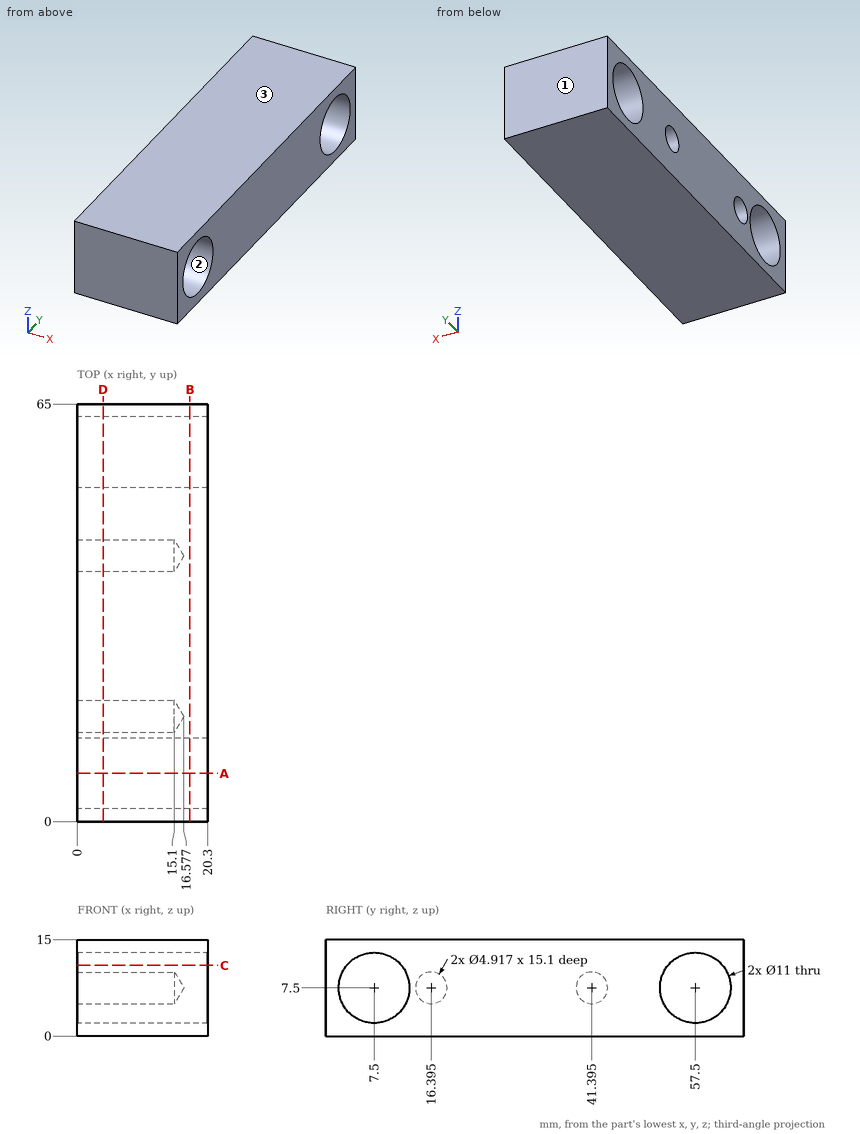
Answer from the drawing. Dimensions are ordinates in mm from the lowest x, y and z of the part. Coordinates: 2 decimals unless noted, no trailing zeros. Loops run counter-clockwise (first coordinate to the right, second up) from the corner with the lowest first, then second, coordinate; pieces in that order, holes last. Notation, with made-up numbers: (69, -1.75) -> (100, -1.75) arc R31 ccw to (100, 25.25) -> close; hole circle Ø2 at (-36.5, 13.5). An arc over 180 degrees is marked (long way). Return JSON: item names as keys, results as strings.
Item 1: Find section D-D (x = 4). Determine the outline of the cut face in (y, z) (1 decimal), plus the area to 3 significant figures.
Answers:
{"outline": "(0, 0) -> (65, 0) -> (65, 15) -> (0, 15) -> close; hole circle Ø11 at (7.5, 7.5); hole circle Ø4.9 at (16.4, 7.5); hole circle Ø4.9 at (41.4, 7.5); hole circle Ø11 at (57.5, 7.5)", "area": "747 mm2"}
Item 2: Find section A-A (y = 7.5). Determine the outline of the cut face in (x, z), plus the area to 3 significant figures.
Answers:
{"outline": "(0, 0) -> (20.3, 0) -> (20.3, 2) -> (0, 2) -> close; (0, 13) -> (20.3, 13) -> (20.3, 15) -> (0, 15) -> close", "area": "81.2 mm2"}
Item 3: Flat-ended cylindrical pins translate along their axes: P1, Ø1, axis at y = 27.5, z = 13, coming from the -X side; P2, Ø6.5, axis at y = 57.5, z = 7.5, coming from the -X side. Find the tip coordinate at first contact, or state that the pin passes through.
Answers:
{"P1": "stops at x = 0", "P2": "passes through"}
Item 4: Find section B-B (x = 17.5). Determine the outline of the cut face in (y, z), plus the area to 3 significant figures.
Answers:
{"outline": "(0, 0) -> (65, 0) -> (65, 15) -> (0, 15) -> close; hole circle Ø11 at (7.5, 7.5); hole circle Ø11 at (57.5, 7.5)", "area": "785 mm2"}
Item 5: Find section C-C (z = 11). Determine the outline of the cut face in (x, y).
Answers:
{"outline": "(0, 0) -> (20.3, 0) -> (20.3, 3.26) -> (0, 3.26) -> close; (0, 11.74) -> (20.3, 11.74) -> (20.3, 53.26) -> (0, 53.26) -> close; (0, 61.74) -> (20.3, 61.74) -> (20.3, 65) -> (0, 65) -> close"}
Item 6: Find the intervals of material crossed by probe 1 along Y at (x, z) = (12.5, 7.5); probe 2 along Y at (x, z) = (12, 10.5); probe 3 along Y at (x, z) = (6, 5.75) (1 decimal), in increasing order.
Answers:
{"probe 1": "y = 0 to 2, 13 to 13.94, 18.85 to 38.94, 43.85 to 52, 63 to 65", "probe 2": "y = 0 to 2.89, 12.11 to 52.89, 62.11 to 65", "probe 3": "y = 0 to 2.3, 12.7 to 14.7, 18.1 to 39.7, 43.1 to 52.3, 62.7 to 65"}
Item 7: For a pull along Z with two mould halves and no side action, classify the marked faces 1, 2 and 3 as +Z half, -Z half, draft (parallel to the pull), parting line (faces both ways), or undercut.
Answers:
{"face 1": "draft", "face 2": "undercut", "face 3": "+Z half"}
